CAD build for the part. Positions are in the model's coordinates, mm. A direction names the side the tool comes from. Give positions to 0.01 mm unless a question says otherwise; leave off trailing zeros. Loops run counter-clockwise (first coordinate to the right, second up) from the corner with the lowest first, then second, coordinate; pieces in that order, holes last. Notation, with made-up numbers: M 57.5,79 L 103.5,79 A24 ccw 103.5,114 Z; hole C 15,42 d11. An arc over 180 degrees is marked long. One line per question, with ' | ' between items.
```python
from build123d import *

# Parameters (mm, degrees)
F0_W       = 82.0303186774
F0_H       = 128.9077922702
F0_W_2     = 61.4851098508
F0_H_2     = 52.307818085
F1_DEPTH   = 25.4
F3_DEPTH   = 103.3353582025
F4_W       = 9.9767372012
F4_H       = 6.5656021893
F4_W_2     = 10.380640626
F4_H_2     = 6.5844875485
F5_DEPTH   = 10.1564340293
F6_W       = 10.2968784049
F6_H       = 6.4595692515
F7_W       = 9.5716901124
F7_H       = 6.5711081684
F8_DEPTH   = 7.9249968985
F9_W       = 8.5524487155
F9_H       = 5.1620816675
F9_W_2     = 7.9160258174
F9_H_2     = 5.1903103754
F10_DEPTH  = 1.3433820568
F11_W      = 7.7443979681
F11_H      = 4.5824625995
F11_W_2    = 7.4055045843
F12_DEPTH  = 0.893893186
F14_DEPTH  = 2.8803441674
F15_R      = 5.0749608974
F1_FACE2_W = 52.307818085
F1_FACE2_H = 25.4
F16_DEPTH  = 3.2730977982
F17_W      = 2.0163990557
F17_H      = 9.5695778728
F18_DEPTH  = 23.3533121645


with BuildPart() as f1:
    # F0 (on Top) → F1 (new body)
    with BuildSketch(Plane.XY):
        with Locations((8.9795850217, -5.5929608643)):
            Rectangle(F0_W, F0_H)
        with Locations((10.0128157064, 26.1539090425)):
            Rectangle(F0_W_2, F0_H_2, mode=Mode.SUBTRACT)
    extrude(amount=F1_DEPTH)

    # F2 (on face) → F3 (cut)
    with BuildSketch(Plane(origin=(-32.035574317, 0, 0), x_dir=(0, -1, 0), z_dir=(-1, 0, 0))):
        Polygon((70.0468569994, 4.5824625995), (70.0468569994, 20.2553160489), (24.9904096127, 20.1640632004), (12.1657857671, 4.5824625995), align=None)
    extrude(amount=-F3_DEPTH, mode=Mode.SUBTRACT)

    # F4 (on face) → F5 (join)
    with BuildSketch(Plane(origin=(-32.035574317, 0, 0), x_dir=(0, -1, 0), z_dir=(-1, 0, 0))):
        with Locations((-40.8467017114, 28.6828010947)):
            Rectangle(F4_W, F4_H)
        with Locations((-14.4690144807, 28.6922437742)):
            Rectangle(F4_W_2, F4_H_2)
    extrude(amount=-F5_DEPTH)

    # F6 (on face) + F7 (on face) → F8 (join)
    with BuildSketch(Plane.YZ.offset(49.9947443604)):
        with Locations((15.0959282182, 28.6297846258)):
            Rectangle(F6_W, F6_H)
    with BuildSketch(Plane.YZ.offset(49.9947443604)):
        with Locations((41.0959366709, 28.6855540842)):
            Rectangle(F7_W, F7_H)
    extrude(amount=-F8_DEPTH)

    # F9 (on face) → F10 (join)
    with BuildSketch(Plane.YZ.offset(49.9947443604)):
        with Locations((-57.180442793, 22.8189591662)):
            Rectangle(F9_W, F9_H)
        with Locations((-43.5606203973, 22.8048448123)):
            Rectangle(F9_W_2, F9_H_2)
    extrude(amount=F10_DEPTH)

    # F11 (on face) → F12 (join)
    with BuildSketch(Plane.YZ.offset(49.9947443604)):
        with Locations((-57.1476463228, 2.2912312998)):
            Rectangle(F11_W, F11_H)
        with Locations((-43.6765104532, 2.2912312998)):
            Rectangle(F11_W_2, F11_H)
    extrude(amount=F12_DEPTH)

    # F13 (on face) → F14 (join)
    with BuildSketch(Plane(origin=(-32.035574317, 0, 0), x_dir=(0, -1, 0), z_dir=(-1, 0, 0))):
        with BuildLine():
            Line((24.9904096127, 20.1640632004), (29.7919796658, 20.1737878229))
            ThreePointArc((29.7919796658, 20.1737878229), (22.9361613671, 24.5040209985), (21.9390430586, 16.4567283495))
            Line((21.9390430586, 16.4567283495), (24.9904096127, 20.1640632004))
        make_face()
        with BuildLine():
            ThreePointArc((21.9390430586, 16.4567283495), (27.0402619522, 15.8220273956), (29.7919895134, 20.1640632004))
            ThreePointArc((29.7919895134, 20.1640632004), (29.7919870515, 20.1689255141), (29.7919796658, 20.1737878229))
            Line((29.7919796658, 20.1737878229), (24.9904096127, 20.1640632004))
            Line((24.9904096127, 20.1640632004), (21.9390430586, 16.4567283495))
        make_face()
    extrude(amount=F14_DEPTH)

    # F15 (on face) + F1_face2 (on face) → F16 (join)
    with BuildSketch(Plane.YZ.offset(49.9947443604)):
        with Locations((-24.9904096127, 20.1640632004)):
            Circle(F15_R)
    with BuildSketch(Plane(origin=(-20.729739219, 26.1539090425, 12.7), x_dir=(0, 1, 0), z_dir=(1, 0, 0))):
        Rectangle(F1_FACE2_W, F1_FACE2_H)
    extrude(amount=F16_DEPTH)

    # F17 (on face) → F18 (join)
    with BuildSketch(Plane(origin=(0, 0, 0), x_dir=(1, 0, 0), z_dir=(0, 0, -1))):
        with Locations((51.0029438883, -27.9941596091)):
            Rectangle(F17_W, F17_H)
    extrude(amount=-F18_DEPTH)


solid = f1.part
```
Item 1: Saw through at A-A on y = 25.5. Give the cut face in (x, z).
Conclusion:
outline: M -32.04,0 L -17.46,0 L -17.46,25.4 L -32.04,25.4 Z; M 40.76,0 L 52.01,0 L 52.01,23.35 L 49.99,23.35 L 49.99,25.4 L 40.76,25.4 Z
Item 2: 3-axis set-ups, long thin cutter, end or side, ignore diameter. For faces 1 (the flat face through (50.889, -57, 2)), 2 (the flat face through (46, 9.947, 29)): which of +Z, -Z, +X, -X, +Y, -Y reach the whole face in a straight line?
Conclusion:
face 1: -Z, +X, -Y | face 2: +Z, +X, -Y
Item 3: Drop flat-ended pins along their axis: P1, Ø3.5, axis at x = -25, z = 29.5, coming from the -Y side; P2, Ø8, axis at x = -28, y = 41.5, coming from the +Z side; P3, Ø2.5, axis at y = -56.5, z = 2, coming from the +X side; P4, Ø8, axis at x = 1, z = 17.5, coming from the -Y side. Give the stop position or say it passes through.
Conclusion:
P1: y = 9.28 | P2: z = 31.97 | P3: x = 50.89 | P4: y = -70.05
Item 4: Mould opens along Y. For faces 3 (the flat face through (-32.036, 8, 12)), 4 (the flat face through (46, 20.244, 29)), 5 (the flat face through (8.405, -18.668, 12.482)) say: pulls with the +Y half, pulls with the -Y half, needs draft (parallel to the pull), parting line crosses it, or undercut.
Conclusion:
face 3: needs draft | face 4: undercut | face 5: pulls with the -Y half
Item 5: Saw through at C-C on x = -27. Give the cut face in (y, z).
Conclusion:
outline: M -70.05,0 L 58.86,0 L 58.86,25.4 L 45.84,25.4 L 45.84,31.97 L 35.86,31.97 L 35.86,25.4 L 19.66,25.4 L 19.66,31.98 L 9.28,31.98 L 9.28,25.4 L -70.05,25.4 L -70.05,20.26 L -24.99,20.16 L -12.17,4.58 L -70.05,4.58 Z
Item 6: Saw through at B-B on z = 29.5. Give the cut face in (x, y).
Conclusion:
outline: M -32.04,9.28 L -21.88,9.28 L -21.88,19.66 L -32.04,19.66 Z; M -32.04,35.86 L -21.88,35.86 L -21.88,45.84 L -32.04,45.84 Z; M 42.07,9.95 L 49.99,9.95 L 49.99,20.24 L 42.07,20.24 Z; M 42.07,36.31 L 49.99,36.31 L 49.99,45.88 L 42.07,45.88 Z
Item 7: Drill centre lines: line 1 along X through (y, z) = (16, 28); line 2 along X through (y, z) = (51, 14.5); line 3 along Z through (x, y) = (41, -63). Where is each one in solid material? Low to high. Write a range as [from, to].
Conclusion:
line 1: [-32.04, -21.88], [42.07, 49.99] | line 2: [-32.04, -17.46], [40.76, 49.99] | line 3: [0, 4.58], [20.24, 25.4]
Item 8: Saw through at D-D on x = -9. Give the cut face in (y, z).
Conclusion:
outline: M -70.05,0 L 0,0 L 0,25.4 L -70.05,25.4 L -70.05,20.26 L -24.99,20.16 L -12.17,4.58 L -70.05,4.58 Z; M 52.31,0 L 58.86,0 L 58.86,25.4 L 52.31,25.4 Z
